Work out the finished part from the listing and answer in its coordinate system (mm). A direction names the side the tool comes from. Round coordinates to 2 decimals unless told otherwise and drop trailing zeros. Order: outer loops, then holes, each group sorted by start corner. A loop starts at its lowest first (then second) coordinate and runs counter-clockwise, first axis right, second up. Notation, with made-up numbers: M 77.25,0 L 110.25,0 A29 ccw 110.25,23 Z; hole C 20,30.25 d3. An arc over 180 degrees is marked long. Return JSON: item names as keys, results as strings.
from build123d import *

# Parameters (mm, degrees)
F0_R     = 6.5
F1_DEPTH = 80
F2_R     = 1.6
F4_DEPTH = 1.2
F6_DEPTH = 100


with BuildPart() as f1:
    # F0 (on Right) → F1 (new body)
    with BuildSketch(Plane.YZ):
        with BuildLine():
            ThreePointArc((-8.9, -4.8), (-6.29325, -11.09325), (0, -13.7))
            Line((0, -13.7), (85.2, -13.7))
            ThreePointArc((85.2, -13.7), (91.49325, -11.09325), (94.1, -4.8))
            Line((94.1, -4.8), (94.1, 11))
            ThreePointArc((94.1, 11), (93.611063, 13.015835), (92.252914, 14.583662))
            ThreePointArc((92.252914, 14.583662), (84.791152, 8.311781), (78.1, 15.4))
            ThreePointArc((78.1, 15.4), (71, 8.3), (63.9, 15.4))
            ThreePointArc((63.9, 15.4), (56.8, 8.3), (49.7, 15.4))
            ThreePointArc((49.7, 15.4), (42.6, 8.3), (35.5, 15.4))
            ThreePointArc((35.5, 15.4), (28.4, 8.3), (21.3, 15.4))
            ThreePointArc((21.3, 15.4), (14.2, 8.3), (7.1, 15.4))
            ThreePointArc((7.1, 15.4), (0.408848, 8.311781), (-7.052914, 14.583662))
            ThreePointArc((-7.052914, 14.583662), (-8.411063, 13.015835), (-8.9, 11))
            Line((-8.9, 11), (-8.9, -4.8))
        make_face()
        Circle(F0_R, mode=Mode.SUBTRACT)
        with Locations((14.2, 0)):
            Circle(F0_R, mode=Mode.SUBTRACT)
        with Locations((28.4, 0)):
            Circle(F0_R, mode=Mode.SUBTRACT)
        with Locations((42.6, 0)):
            Circle(F0_R, mode=Mode.SUBTRACT)
        with Locations((56.8, 0)):
            Circle(F0_R, mode=Mode.SUBTRACT)
        with Locations((71, 0)):
            Circle(F0_R, mode=Mode.SUBTRACT)
        with Locations((85.2, 0)):
            Circle(F0_R, mode=Mode.SUBTRACT)
    extrude(amount=F1_DEPTH)

    # F2
    f2_edges = [f1.edges().sort_by_distance(p)[0] for p in [
        (40, 78.1, 15.4),
        (40, 63.9, 15.4),
        (40, 49.7, 15.4),
        (40, 35.5, 15.4),
        (40, 21.3, 15.4),
        (40, 7.1, 15.4),
        (40, 92.252914, 14.583662),
        (40, -7.052914, 14.583662),
    ]]
    fillet(f2_edges, radius=F2_R)

    # F3 (on face) → F4 (join)
    with BuildSketch(Plane(origin=(0, 0, 0), x_dir=(0, -1, 0), z_dir=(-1, 0, 0))):
        with BuildLine():
            ThreePointArc((-92.5, 12.267136), (-93.631371, 11.798507), (-94.1, 10.667136))
            Line((-94.1, 10.667136), (-94.1, -4.8))
            ThreePointArc((-94.1, -4.8), (-91.49325, -11.09325), (-85.2, -13.7))
            Line((-85.2, -13.7), (0, -13.7))
            ThreePointArc((0, -13.7), (6.29325, -11.09325), (8.9, -4.8))
            Line((8.9, -4.8), (8.9, 10.667136))
            ThreePointArc((8.9, 10.667136), (8.431371, 11.798507), (7.3, 12.267136))
            Line((7.3, 12.267136), (-92.5, 12.267136))
        make_face()
    extrude(amount=F4_DEPTH)

    # F5 (on Front) → F6 (cut, symmetric)
    with BuildSketch(Plane.XZ):
        Polygon((79.8, -13.7), (-1.2, -8.4), (-2.687202, -26.329059), (79.8, -25.427904), align=None)
    extrude(amount=F6_DEPTH, both=True, mode=Mode.SUBTRACT)


solid = f1.part
Item 1: Consider line 1 along X through (y, z) = (2.5, -5.5); line 2 along Z through (x, y) = (66.5, 9); line 3 along Z through (x, y) = (18, 74). Determine where each line is inside the solid, lowest interval first. Write a range as [from, to].
Output:
{"line 1": "x = [-1.2, 0]", "line 2": "z = [-12.83, -3.9], [3.9, 10.57]", "line 3": "z = [-9.66, -5.77], [5.77, 8.96]"}
Item 2: Find section D-D (y = 43). Determine the outline of the cut face in (x, z), plus the area to 3 significant figures.
Output:
{"outline": "M -1.2,-8.4 L 79.8,-13.7 L 80,-13.7 L 80,-6.49 L 0,-6.49 L 0,6.49 L 80,6.49 L 80,8.31 L 0,8.31 L 0,12.27 L -1.2,12.27 Z", "area": "539 mm^2"}
Item 3: Which of the six approach directions +Z, -Z, +X, -X, +Y, -Y give full straight-line access (tool end or side, diameter ignored) to faces 1 (the flat face through (0, 43, 0)), 2 (the cylindrical face through (48.991, -8.024, -8.65)), 3 (the cylindrical face through (39.4, 14.3, 8.3))?
Output:
{"face 1": "+X", "face 2": "-Z, +X, -X, -Y", "face 3": "+Z, +X"}
Item 4: The mould has two halves that part along Y. Classify faces 4 (the cylindrical face through (39.44, 78.706, 0.286)), 5 (the flat face through (0, 71, 0)), 6 (the flat face through (80, 42, -9)), 7 (the flat face through (40, 94.1, 3)): pulls with the +Y half, pulls with the -Y half, needs draft (parallel to the pull), parting line crosses it, or undercut.
Output:
{"face 4": "undercut", "face 5": "undercut", "face 6": "needs draft", "face 7": "pulls with the +Y half"}
Item 5: Find section A-A (y = 71). Determine the outline of the cut face in (x, z), plus the area to 3 significant figures.
Output:
{"outline": "M -1.2,-8.4 L 79.8,-13.7 L 80,-13.7 L 80,-6.5 L 0,-6.5 L 0,6.5 L 80,6.5 L 80,8.3 L 0,8.3 L 0,12.27 L -1.2,12.27 Z", "area": "537 mm^2"}
Item 6: Find section C-C (x = 5). State how many separate pieces and enclosed holes the cut face has, plus the area to 3 significant figures.
Output:
{"separate pieces": "1", "enclosed holes": "7", "area": "980 mm^2"}
Item 7: Each of these flat-tipped pins is pushed along its axis until it touches: pin 1 (10.5 mm diameter, centred on y = 14.2, z = 0, fed in from +X); pin 2 (2 mm diameter, centred on x = 39, z = -8, fed in from +Y); pin 3 (2 mm diameter, centred on x = 60, z = -10.5, fed in from +Y). Where does it stop, or does it pass through?
Output:
{"pin 1": "stops at x = 0", "pin 2": "stops at y = 93.82", "pin 3": "stops at y = 92.76"}
